```python
from build123d import *

# Parameters (mm, degrees)
SKETCH_1_R      = 2.5
EXTRUDE_1_DEPTH = 100
EXTRUDE_2_DEPTH = 3
EXTRUDE_START   = 100
EXTRUDE_3_DEPTH = 3


with BuildPart() as part:
    # 草圖1 → 填料-伸長1 (new body)
    with BuildSketch(Plane.XY):
        Circle(SKETCH_1_R)
    extrude(amount=EXTRUDE_1_DEPTH)

    # 草圖3 → 填料-伸長2 (add)
    with BuildSketch(Plane.XY):
        Polygon((2.020725942, 3.5), (-2.020725942, 3.5), (-4.041451884, 0), (-2.020725942, -3.5), (2.020725942, -3.5), (4.041451884, 0), align=None)
    extrude(amount=-EXTRUDE_2_DEPTH)

    # 草圖4 → 填料-伸長3 (add)
    with BuildSketch(Plane.XY.offset(EXTRUDE_START)):
        Polygon((-4.041451884, 0), (-2.020725942, -3.5), (2.020725942, -3.5), (4.041451884, 0), (2.020725942, 3.5), (-2.020725942, 3.5), align=None)
    extrude(amount=EXTRUDE_3_DEPTH)


solid = part.part
```
Read the model definition and answer for the solid it produces. Units are mm, in the model's axes. A direction names the side the tool comes from. Coordinates: 2 decimals unless noted, no trailing zeros. Write each loop counter-clockwise with the first axis right and the second up, starting at its lowest first coordinate (ties: lowest second). Pieces come first, ordered by that corner, then holes. Notation, with made-up numbers: (18.25, -36.5) -> (26.25, -36.5) arc R31 ccw to (26.25, -2.5) -> close; hole circle Ø8 at (4.25, 33.5). An arc over 180 degrees is marked (long way). Write item = value, one per line.
(1) For a pull along Z with two mould halves and no side action, classify faces 1 (the face through (3, 0, 100)), 2 (the face through (-3.045, -1.726, -1.479)), 3 (the face through (-0.54, -2.44, 49.3)), 4 (the face through (0, 0, -3)) as +Z half, -Z half, draft (parallel to the pull), parting line (faces both ways), or undercut.
From the geometry:
face_1 = undercut
face_2 = draft
face_3 = undercut
face_4 = -Z half
(2) Section A-A on y = -1.25 is taken. Write down the section's boundary in (x, z).
From the geometry:
outline = (-3.32, -3) -> (3.32, -3) -> (3.32, 0) -> (2.17, 0) -> (2.17, 100) -> (3.32, 100) -> (3.32, 103) -> (-3.32, 103) -> (-3.32, 100) -> (-2.17, 100) -> (-2.17, 0) -> (-3.32, 0) -> close
(3) Section B-B on x = 0 is taken. Write down the section's boundary in (y, z), plus the area to 3 significant figures.
From the geometry:
outline = (-3.5, -3) -> (3.5, -3) -> (3.5, 0) -> (2.5, 0) -> (2.5, 100) -> (3.5, 100) -> (3.5, 103) -> (-3.5, 103) -> (-3.5, 100) -> (-2.5, 100) -> (-2.5, 0) -> (-3.5, 0) -> close
area = 542 mm2
(4) Which of the six approach directions +Z, -Z, +X, -X, +Y, -Y give full straight-line access (tool end or side, diameter ignored) to faces 5 (the face through (-3, 1.8, -1.5)), 6 (the face through (3, 0, 0))?
From the geometry:
face_5 = +Z, -Z, -X, +Y
face_6 = none
(5) Straight lines are drawn through the part: L1, parallel to Z at x = -3, y = 0.5; L2, parallel to X at y = -0.25, z = 7; L3, parallel to X at y = 1, z = 57.5. For each, find the intervals that lie inside material, in ascending order. Write a range as from..to.
From the geometry:
L1 = -3..0, 100..103
L2 = -2.49..2.49
L3 = -2.29..2.29
(6) Section C-C on z = 91.5 is taken. Write down the section's boundary in (x, y).
From the geometry:
outline = circle Ø5 at (0, 0)
(7) Given pin 1 Ø4 at (x, z) = (-2.5, 84) entering from +Y; pin 2 Ø4 at (x, z) = (-1, 10) entering from +Y; pin 3 Ø1.5 at (x, z) = (-2.5, 78.5) entering from -Y, each flat-ended and moving along its own axis, determine where each tip first touches the part or whether it passes through.
From the geometry:
pin_1 = 2.45
pin_2 = 2.5
pin_3 = -1.79
